Could you check a few things on this model? Use its own coordinates, in mm. A direction names the side the tool comes from. Round coordinates to 2 decimals unless told otherwise and drop trailing zeros. Loops run counter-clockwise (first coordinate to the right, second up) from the corner with the lowest first, then second, coordinate; pieces in that order, holes last. Notation, with made-up numbers: (47.25, 66.5) -> (63.25, 66.5) arc R35 cw to (63.25, 100.5) -> close; hole circle Ø2 at (62, -40). An arc over 180 degrees is marked (long way). Put each result on its own line as item: value. Start each with the question number.
1. Imagine slicing it at A-A, the plane x = 0. Please give me the cut outline in (y, z).
2. If we mould it in two halves opening along X, with no side actions, what happens to faces 1 (the cylindrical face through (1.213, -29.475, 1.74)), 2 (the cylindrical face through (-13.926, 15.004, 0.986))? For each: pulls with the +X half, pulls with the -X half, needs draft (parallel to the pull), parting line crosses it, or undercut.
3. Which directions (+Z, -Z, +X, -X, +Y, -Y) give clear straight access to the entire face, cutting with the end or side of a thin tool? Please do faces 3 (the flat face through (17, 14, 2)), 4 (the cylindrical face through (17.074, 15.004, 0.986)), 5 (the flat face through (-6, 28, 2)).
4. Imagine slicing it at C-C, the plane y = 15.5. Count the separate pieces of the cut face and the enclosed holes in it, and give its area (3 significant figures).
5. Imagine slicing it at B-B, the plane y = 0. Please give me the cut outline in (x, z), and give its area (3 significant figures).
6. I need wall thicknesses on line 1 (Y direction, x = 1.5, z = 1.05); line 2 (X direction, y = 15.5, z = 0.95); line 3 (X direction, y = -15.5, z = 1.3). Which ranges of each line are inside material? Lowest first, please. Write a range as [from, to].
7. I'm going to push flat-ended pins straight in: P1, Ø1.5, axis at x = -11.5, z = 0.5, coming from the -Y side; P2, Ø4.5, axis at x = -25, y = 0, coming from the +Z side; P3, Ø1.5, axis at y = 20, z = 3, coming from the +X side. Where does each tip first touch, or does it pass through?
Autodesk Inventor part; units mm, degrees
ref_plane "YZ Plane" through (0, 0, 0) normal (1, 0, 0) x (0, 1, 0)
ref_plane "XZ Plane" through (0, 0, 0) normal (0, 1, 0) x (-1, 0, 0)
ref_plane "XY Plane" through (0, 0, 0) normal (0, 0, 1) x (1, 0, 0)
sketch "Sketch1" plane through (0, 0, 0) normal (0, 0, 1) x (1, 0, 0)
  circle A0 centre (0, 0) radius 29.5
  line L0 (-15.5, -15.5) -> (15.5, -15.5) construction
  line L1 (15.5, -15.5) -> (15.5, 15.5) construction
  line L2 (15.5, 15.5) -> (-15.5, 15.5) construction
  line L3 (-15.5, 15.5) -> (-15.5, -15.5) construction
  line L4 (-15.5, -15.5) -> (15.5, 15.5) construction
  line L5 (15.5, -15.5) -> (-15.5, 15.5) construction
  circle A1 centre (-15.5, 15.5) radius 1.65
  circle A2 centre (15.5, 15.5) radius 1.65
  circle A3 centre (15.5, -15.5) radius 1.65
  circle A4 centre (-15.5, -15.5) radius 1.65
  circle A5 centre (0, 0) radius 11.5
  line L6 (0, 0) -> (25, 0) construction
  circle A6 centre (0, 0) radius 25 construction
  circle A7 centre (25, 0) radius 1.65
  circle A8 centre (-25, 0) radius 1.65
  circle A9 centre (0, -25) radius 1.65
  line L7 (-25, 0) -> (0, 0) construction
  line L8 (0, 0) -> (0, -25) construction
  dimension "d0" = 59
  dimension "d1" = 3.3
  dimension "d2" = 23
  dimension "d3" = 31
  dimension "d4" = 50
  dimension "d5" = 3.3
extrude "Extrusion1" add sketch "Sketch1" along normal blind 3.5
sketch "Sketch2" plane through (0, 0, 3.5) normal (0, 0, 1) x (1, 0, 0)
  circle A0 centre (0, -25) radius 1.65
  circle A1 centre (0, -25) radius 3
  circle A2 centre (25, 0) radius 1.65
  circle A3 centre (25, 0) radius 3
  circle A4 centre (-25, 0) radius 1.65
  circle A5 centre (-25, 0) radius 3
  circle A6 centre (-15.5, -15.5) radius 1.65
  circle A7 centre (-15.5, -15.5) radius 3
  circle A8 centre (15.5, -15.5) radius 1.65
  circle A9 centre (15.5, -15.5) radius 3
  circle A10 centre (15.5, 15.5) radius 1.65
  circle A11 centre (15.5, 15.5) radius 3
  circle A12 centre (-15.5, 15.5) radius 1.65
  circle A13 centre (-15.5, 15.5) radius 3
  point P0 (0, 0)
  dimension "d8" = 6
extrude "Extrusion2" cut sketch "Sketch2" against normal blind 1.5 contours A0 | A1 | A2 | A3 | A4 | A5 | A6 | A7 | A8 | A9 | A10 | A11 | A12 | A13
sketch "Sketch3" plane through (0, 0, 3.5) normal (0, 0, 1) x (1, 0, 0)
  line L0 (0, 31.5) -> (0, 27.5) construction
  circle A0 centre (0, 0) radius 29.5 construction
  line L1 (-6, 31.5) -> (-6, 27.5)
  line L2 (6, 27.5) -> (6, 31.5)
  arc A1 (6, 31.5) -> (-6, 31.5) centre (0, 31.5) ccw
  arc A2 (-6, 27.5) -> (6, 27.5) centre (0, 27.5) ccw
  point P0 (0, 29.5)
  dimension "d14" = 2
  dimension "d15" = 6
extrude "Extrusion3" cut sketch "Sketch3" against normal through all
chamfer "Chamfer1" distance 1 angle 45 2 edges at (0, -29.5, 3.5) (0, -29.5, 0)
properties part number "WristMotorPlate"
Entries:
1. outline: (-29.5, 1) -> (-28.5, 0) -> (-26.65, 0) -> (-26.65, 2) -> (-28, 2) -> (-28, 3.5) -> (-28.5, 3.5) -> (-29.5, 2.5) -> close; (-23.35, 0) -> (-11.5, 0) -> (-11.5, 3.5) -> (-22, 3.5) -> (-22, 2) -> (-23.35, 2) -> close; (11.5, 0) -> (21.5, 0) -> (21.5, 3.5) -> (11.5, 3.5) -> close
2. face 1: parting line crosses it
2. face 2: undercut
3. face 3: +Z
3. face 4: +Z, -Z
3. face 5: +Z, -Z, +Y
4. separate pieces: 3
4. enclosed holes: 0
4. area: 142 mm^2
5. outline: (-29.5, 1) -> (-28.5, 0) -> (-26.65, 0) -> (-26.65, 2) -> (-28, 2) -> (-28, 3.5) -> (-28.5, 3.5) -> (-29.5, 2.5) -> close; (-23.35, 0) -> (-11.5, 0) -> (-11.5, 3.5) -> (-22, 3.5) -> (-22, 2) -> (-23.35, 2) -> close; (11.5, 0) -> (23.35, 0) -> (23.35, 2) -> (22, 2) -> (22, 3.5) -> (11.5, 3.5) -> close; (26.65, 0) -> (28.5, 0) -> (29.5, 1) -> (29.5, 2.5) -> (28.5, 3.5) -> (28, 3.5) -> (28, 2) -> (26.65, 2) -> close
5. area: 92.8 mm^2
6. line 1: [-29.46, -25.69], [-24.31, -11.4], [11.4, 21.69]
6. line 2: [-25.04, -17.15], [-13.85, 13.85], [17.15, 25.04]
6. line 3: [-25.1, -17.15], [-13.85, 13.85], [17.15, 25.1]
7. P1: y = -27.4
7. P2: z = 2
7. P3: x = 22.19
